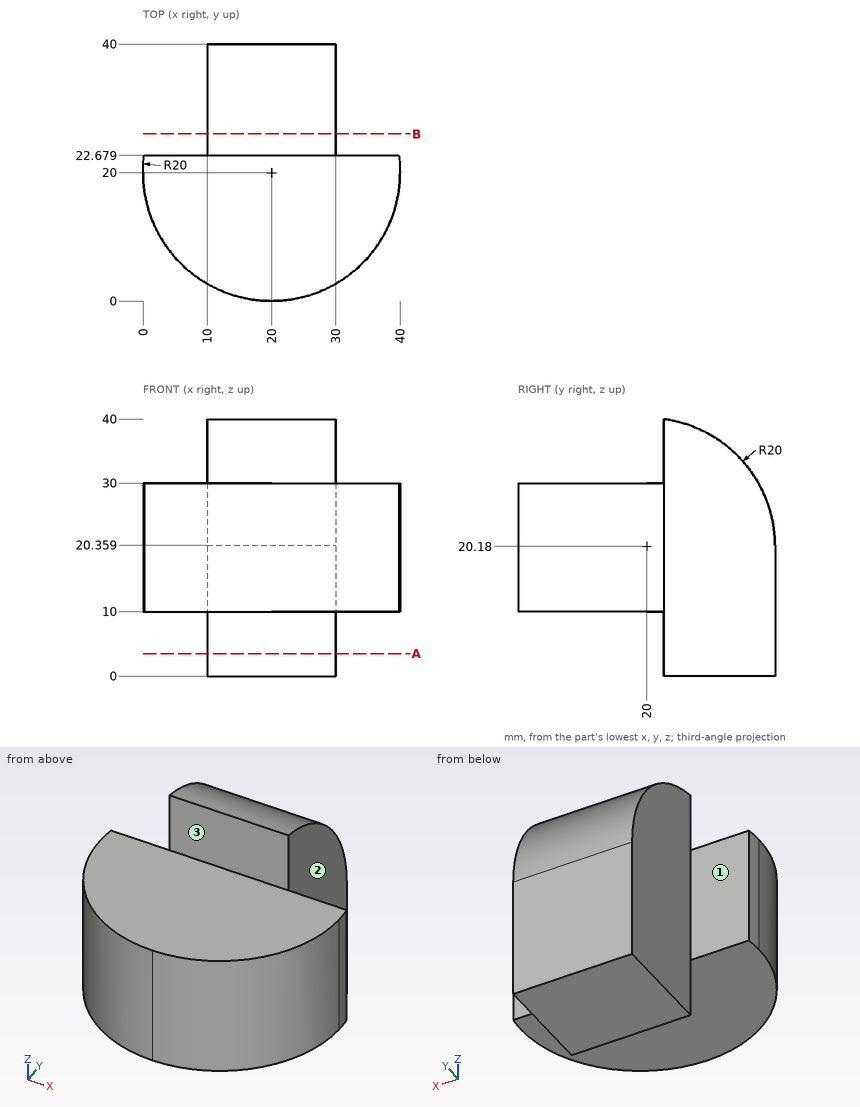
Study the drawing (mm; zero at the part's minimum x, y, z) and answer. A direction names the side the tool comes from. Give positions to 0.01 mm unless a question says otherwise; leave off trailing zeros. Write each loop counter-clockwise with the first axis right and the second up, starting at its lowest first coordinate (ties: lowest second). Pieces come first, ordered by that corner, then holes. Notation, with made-up numbers: (-1.5, -4.5) - (20.5, -4.5) arc R31 ccw to (20.5, 27.5) - close; hole circle Ø8 at (-2, 57.25). An arc over 180 degrees is marked (long way). One line per question, with ' | ' between items. Start each with the question number.
1. Given P1, Ø3, axis at y = 9, z = 12, coming from the +X side; P2, Ø5, axis at x = 21, y = 11.5, coming from the +Z side; P3, Ø12, axis at x = 34.5, y = 18.5, coming from the -Z side, each flat-ended and moving along its own axis, determine where each tip first touches the part or whether it passes through.
2. For the marked faces 1, 2 and 3, determine the directions among +Z, -Z, +X, -X, +Y, -Y from which every point of the face is accessible in a straight line to the end or side of a thin tool.
3. Straight lines are drawn through the part: line 1 (Z direction, x = 3.5, y = 15); line 2 (Y direction, x = 31.5, z = 16) (1 decimal). For each, find the intervals that lie inside material, in ascending order.
4. Section B-B, the plane y = 26 is taken. Determine the outline of the cut face in (x, z), then the cut area to 3 significant figures.
5. Section A-A, the plane z = 3.5 is taken. Determine the outline of the cut face in (x, y).
Result:
1) P1: stops at x = 37.6 | P2: stops at z = 30 | P3: stops at z = 10
2) face 1: +Z, -Z, -X, +Y | face 2: +Z, -Z, +X, +Y | face 3: +Z, +X, -X, -Y
3) line 1: z = 10 to 30 | line 2: y = 3.6 to 22.7
4) outline: (10, 0) - (30, 0) - (30, 39.26) - (10, 39.26) - close | area: 785 mm2
5) outline: (10, 22.68) - (30, 22.68) - (30, 40) - (10, 40) - close
